The drawing under review shows one solid part. Ordinate dimensions are in mm from its lowest x, y, z. A direction names the side the tool comes from. Round coordinates to 2 decimals unless told otherwise and drop trailing zeros. Order: outer loops, then holes, each group sorted by start corner. A loop starts at its lowest first (then second) coordinate and runs counter-clockwise, first axis right, second up.
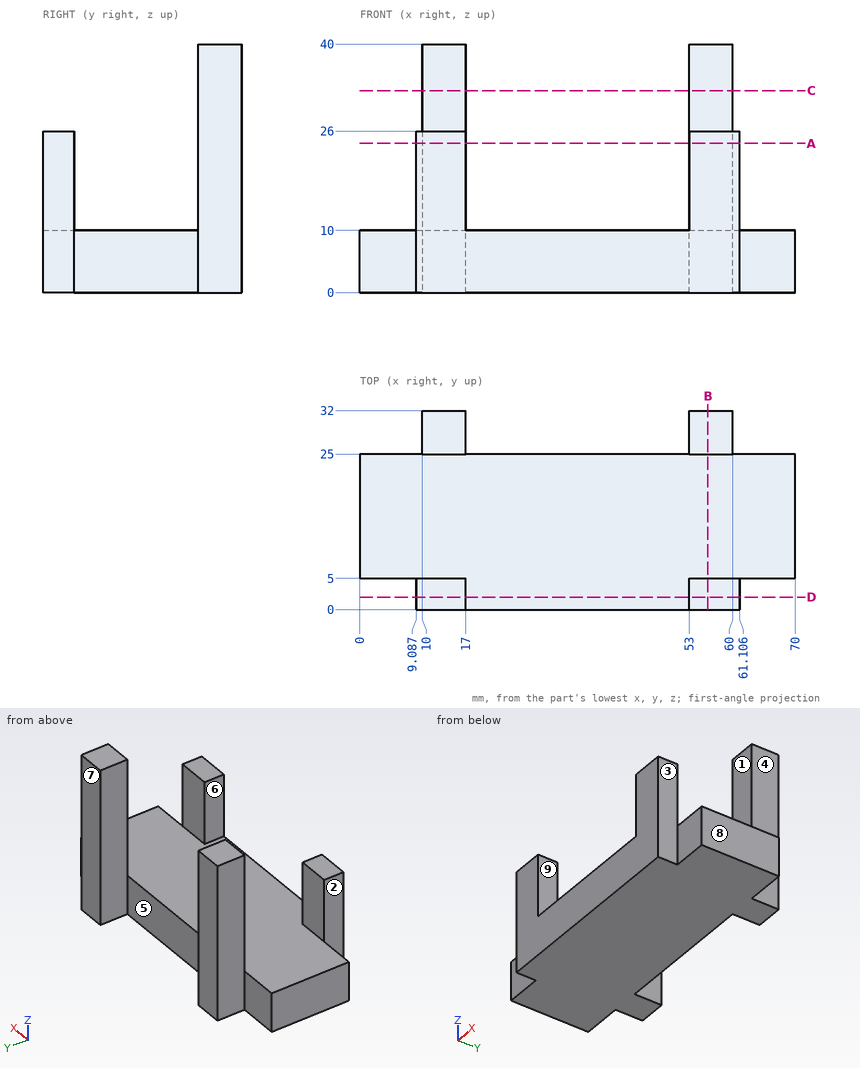
Q1. Mouldability with a two-part tool opening along X and no side actions: class the marked faces 6, 7, 8 and 9 as +X half, -X half, draft (parallel to the pull), parting line (faces both ways), or undercut.
Q2. Take a section at A-A, the plane z = 24. State the section outline as (x, y) points (1 decimal).
Q3. Wall thickness on line 1 (X direction, y = 2, z = 22) (1 decimal); line 2 (Z direction, x = 21.5, y = 7.5); line 3 (Y direction, x = 55, z = 11.5): over which ranges is each line inside the solid? List them lowest first.
Q4. Take a section at B-B, the plane x = 56. State the section outline as (y, z) points, plus the area to 3 significant figures.
Q5. Tool access review of the marked faces 1, 2, 3, 4 and 5: name each direction out of +Z, -Z, +X, -X, +Y, -Y from which nothing blocks a thin tool from reaching the whole face with its end or side.
Q6. Take a section at C-C, the plane z = 32.5. State the section outline as (x, y) points.
Q7. Take a section at D-D, the plane y = 2. State the section outline as (x, z) points (1 decimal).
Q8. Clearance check with flat-ended pins moving along their axes: pin 1 (2 mm diameter, centred on x = 14, z = 28, fed in from -Y); pin 2 (8 mm diameter, centred on x = 4.5, z = 3, fed in from +Y); pin 3 (4 mm diameter, centred on y = 3.5, z = 13, fed in from -X). State where each tip first meets the part, or that it passes through.
Working result:
1. face 6: undercut
1. face 7: draft
1. face 8: +X half
1. face 9: undercut
2. outline: (9.1, 0) - (17, 0) - (17, 5) - (9.1, 5) - close; (10, 25) - (17, 25) - (17, 32) - (10, 32) - close; (53, 0) - (61.1, 0) - (61.1, 5) - (53, 5) - close; (53, 25) - (60, 25) - (60, 32) - (53, 32) - close
3. line 1: x = 9.1 to 17, 53 to 61.1
3. line 2: z = 0 to 10
3. line 3: y = 0 to 5, 25 to 32
4. outline: (0, 0) - (32, 0) - (32, 40) - (25, 40) - (25, 10) - (5, 10) - (5, 26) - (0, 26) - close
4. area: 610 mm2
5. face 1: +Z, +X, -X
5. face 2: +Z, -Z, -X, -Y
5. face 3: +Z, -Z, +X, -Y
5. face 4: +Z, -Z, +X, +Y
5. face 5: +Z, -Z, +Y
6. outline: (10, 25) - (17, 25) - (17, 32) - (10, 32) - close; (53, 25) - (60, 25) - (60, 32) - (53, 32) - close
7. outline: (9.1, 0) - (61.1, 0) - (61.1, 26) - (53, 26) - (53, 10) - (17, 10) - (17, 26) - (9.1, 26) - close
8. pin 1: stops at y = 25
8. pin 2: stops at y = 25
8. pin 3: stops at x = 9.09
